Input: part model. Units: mm. Frame: model coordinates. Face numbers are marked on the shaded views. A direction names the side the tool comes from. Coordinates: 2 decimals unless noted, no trailing zeros. Loops run counter-clockwise (first coordinate to the right, second up) from the corner with the lowest first, then second, coordinate; pieces in that order, holes last. Notation, with made-up numbers: M 14,70.25 L 25,70.25 A17 ccw 25,95.25 Z; hole C 5,-11.75 d6. An arc over 180 degrees is marked long. Use a Markdown table: item, result. Add a question column.
1. Pin query (flat end, axial travel): pin 1 (1 mm diameter, centred on x = 37, y = -43, fed in from -Z); pin 2 (2 mm diameter, centred on x = 105.5, z = 27, fed in from -Y); pin 3 (7 mm diameter, centred on y = -47.73, z = 47.73, fed in from +X); pin 4 (1.5 mm diameter, centred on x = 100, z = -5, fed in from +Y). Return the tip coordinate at first contact, or that it passes through.
2. Section D-D on z = 0. State how many separate pieces and enclosed holes the cut face has, then the cut area to 3 significant figures.
3. Line query: L1, parallel to Z at x = 189, y = -23; L2, parallel to Z at x = 13.5, y = -44.5; L3, parallel to X at y = 25, z = 42.5. Output: solid intervals per line, ascending. Write a range as [from, to].
4. Set-up query: the marked faces 4 and 5. Return all of +Z, -Z, +X, -X, +Y, -Y with unobstructed straight access to the full face (end or side cutting, diameter ignored); none if empty.
5. Section A-A on y = 67.5. Output: boundary loops of the cut face in (x, z), then the cut area to 3 significant figures.
6. Draft query along X for the marked faces 1, 2 and 3. Return one class per face: +X half, -X half, draft (parallel to the pull), parting line (faces both ways), or undercut.
7. Section C-C on x = 108. Output: boundary loops of the cut face in (y, z).
Autodesk Inventor part; units mm, degrees
ref_plane "YZ Plane" through (0, 0, 0) normal (1, 0, 0) x (0, 1, 0)
ref_plane "XZ Plane" through (0, 0, 0) normal (0, 1, 0) x (-1, 0, 0)
ref_plane "XY Plane" through (0, 0, 0) normal (0, 0, 1) x (1, 0, 0)
sketch "Sketch2" plane through (0, 0, 0) normal (0, 0, 1) x (1, 0, 0)
  line L0 (0, 54.5) -> (192, 54.5)
  line L1 (254.7886, 18.124) -> (254.7886, 0) construction
  line L2 (192, 54.5) -> (254.7886, 18.124)
  line L3 (254.7886, 18.124) -> (325.1228, 36.97)
  line L4 (254.7886, 18.124) -> (254.7886, 43.3259) construction
  line L5 (0, 0) -> (254.7886, 0)
  line L6 (325.1228, 36.97) -> (325.1228, 0)
  line L7 (192, 54.5) -> (254.7886, 18.124)
  line L8 (325.1228, 0) -> (305.1228, 0)
  line L9 (-65.0246, 0) -> (390.1474, 0)
  line L10 (0, 57.5) -> (192, 57.5)
  line L11 (193.5039, 57.0958) -> (255.2149, 21.3441)
  line L12 (255.2149, 21.3441) -> (325.1228, 40.0758)
  line L13 (325.1228, 36.97) -> (325.1228, 40.0758)
  line L14 (0, 54.5) -> (0, 57.5)
  line L15 (193.5039, 57.0958) -> (192.8038, 57.5)
  line L16 (193.5039, 57.0958) -> (200.0085, 57.0958) construction
  line L17 (192, 57.5) -> (192.8038, 57.5)
  line L18 (325.1228, 40.0758) -> (325.1228, 57.5)
  line L19 (317.1228, 57.5) -> (317.1228, 37.9322)
  line L20 (325.1228, 0) -> (325.1228, 58.5)
  line L21 (317.1228, 58.5) -> (317.1228, 57.5)
  line L22 (317.1228, 58.5) -> (325.1228, 58.5)
  point P0 (254.7886, 31.9804)
  point P1 (325.1228, 59.5)
  point P2 (321.1228, 58.5)
  dimension "d2" = 18.124
  dimension "d9" = 54.5
  dimension "d43" = 192
  dimension "d76" = 20
  dimension "d141" = 3
  dimension "d142" = 3
  dimension "d143" = 3
  dimension "d144" = 150
  dimension "d159" = 8
  dimension "d199" = 58.5
revolve "Revolution1" add sketch "Sketch2" angle 360 about axis through (0, 0, 0) along (1, 0, 0) contours L14 L10 L17 L15 L11 L12 L13 L3 L2 L0
sketch "Sketch24" plane through (0, 0, 0) normal (-1, 0, 0) x (0, 0, 1)
  circle A0 centre (0, 0) radius 75
  circle A1 centre (0, 0) radius 21.3441
  circle A2 centre (0, 0) radius 57.5
  dimension "d155" = 150
  dimension "d156" = 115
extrude "Extrusion9" add sketch "Sketch24" against normal blind 3 contours A0
revolve "Revolution4" add sketch "Sketch2" angle 360 about axis through (-10, 0, 0) along (1, 0, 0) contours L12 L19 L21 L22 L20 L18
sketch "Sketch25" plane through (0, 0, 0) normal (0, 0, 1) x (1, 0, 0)
  line L0 (317.1228, -54.5) -> (317.1228, 54.5)
  line L1 (317.1228, 54.5) -> (320.1228, 54.5)
  line L2 (317.1228, 54.5) -> (325.1228, 54.5)
  line L3 (320.1228, 54.5) -> (320.1228, 53.5)
  line L4 (320.1228, 53.5) -> (322.1228, 53.5)
  line L5 (322.1228, 53.5) -> (322.1228, 54.5)
  line L6 (322.1228, 54.5) -> (320.7933, 54.5)
  line L7 (317.1228, -58.5) -> (317.1228, 58.5)
  line L8 (317.1228, 54.5) -> (317.1228, 58.5)
  line L9 (320.1189, 58.348) -> (320.0429, 56.8499)
  line L10 (317.1228, 58.5) -> (320.1228, 58.5)
  line L11 (317.1228, 58.5) -> (325.1228, 58.5)
  line L12 (320.1228, 58.5) -> (320.0506, 57.0017)
  point P0 (0, 0)
  dimension "d161" = 3
  dimension "d162" = 1
  dimension "d163" = 2
  dimension "d202" = 3
revolve "Revolution5" [suppressed]
sketch "Sketch26" plane through (0, 0, 0) normal (-1, 0, 0) x (0, 0, 1)
  circle A0 centre (0, 0) radius 18.124
  circle A1 centre (0, 0) radius 67.5
  circle A2 centre (0, 67.5) radius 4
  circle A3 centre (-47.7297, 47.7297) radius 4
  circle A4 centre (-67.5, 0) radius 4
  circle A5 centre (-47.7297, -47.7297) radius 4
  circle A6 centre (0, -67.5) radius 4
  circle A7 centre (47.7297, -47.7297) radius 4
  circle A8 centre (67.5, 0) radius 4
  circle A9 centre (47.7297, 47.7297) radius 4
  point P0 (0, 0)
  dimension "d165" = 135
  dimension "d166" = 8
  dimension "d169" = 360
hole "Hole1" at (0, 67.5, 0) at (0, 47.7297, -47.7297) at (0, 0, -67.5) at (0, 47.7297, 47.7297) at (0, 0, 67.5) at (0, -47.7297, -47.7297) at (0, -67.5, 0) at (0, -47.7297, 47.7297) direction (1, 0, 0) diameter 8 end through all
thread "Thread19"
thread "Thread20"
thread "Thread21"
thread "Thread22"
thread "Thread23"
thread "Thread24"
thread "Thread25"
thread "Thread26"
thread "Thread27"
sketch "Sketch27" plane through (0, 0, 0) normal (0, 0, 1) x (1, 0, 0)
  line L0 (317.1228, -58.5) -> (317.1228, 58.5)
  line L1 (317.1228, 58.5) -> (320.1228, 58.5)
  line L2 (317.1228, 58.5) -> (325.1228, 58.5)
  line L3 (320.1228, 58.5) -> (320.1228, 57)
  line L4 (320.1228, 57) -> (322.1228, 57)
  line L5 (322.1228, 57) -> (322.1228, 58.5)
  line L6 (-65.0246, 0) -> (390.1474, 0)
  point P0 (0, 0)
  dimension "d207" = 3
  dimension "d208" = 1.5
  dimension "d209" = 2
revolve "Revolution6" cut sketch "Sketch27" angle 360 about axis through (-10, 0, 0) along (1, 0, 0)
properties part number "aluminium engine" material "Aluminum 6061"
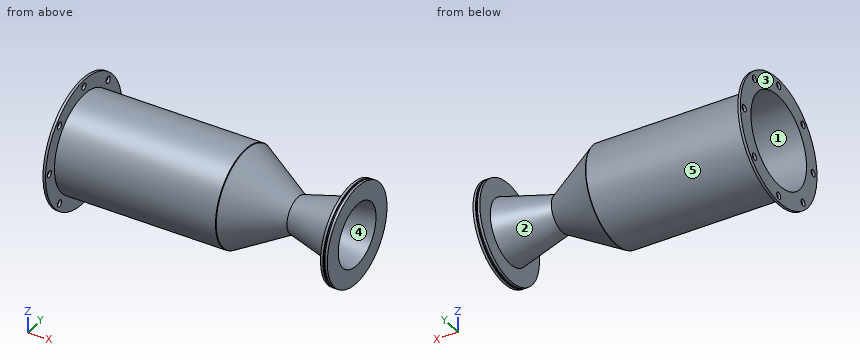
Answers below:
| question | item | result |
|---|---|---|
| 1 | pin 1 | stops at z = -38.73 |
| 1 | pin 2 | stops at y = -51.29 |
| 1 | pin 3 | passes through |
| 1 | pin 4 | stops at y = 57.34 |
| 2 | separate pieces | 4 |
| 2 | enclosed holes | 0 |
| 2 | area | 2,390 mm² |
| 3 | L1 | z = [-52.7, -49.41], [49.41, 52.7] |
| 3 | L2 | z = [-36.41, -31.46], [31.46, 36.41] |
| 3 | L3 | x = [200.96, 206.95], [317.12, 325.12] |
| 4 | face 4 | +X |
| 4 | face 5 | none |
| 5 | outline | M 0,-32.69 L 3,-32.69 L 3,-4 L 0,-4 Z; M 0,4 L 3,4 L 3,32.69 L 0,32.69 Z |
| 5 | area | 172 mm² |
| 6 | face 1 | draft |
| 6 | face 2 | undercut |
| 6 | face 3 | -X half |
| 7 | outline | C 0,0 d115; hole C 0,0 d109 |
